from build123d import *

# Parameters (mm, degrees)
SKETCH2_W                     = 76.2
SKETCH2_H                     = 192
BOSS_EXTRUDE1_DEPTH           = 9.525
M16_CLEARANCE_HOLE1_D         = 17
M4X0_7_TAPPED_HOLE1_D         = 3.3
SKETCH9_R                     = 11.5
CUT_EXTRUDE1_DEPTH            = 179.996240317
FILLET1_SIZE                  = 15
M6X1_0_START                  = -94
M6X1_0_TAPPED_HOLE1_OUTLINE_R = 2.5
M6X1_0_TAPPED_HOLE1_DEPTH     = 12


with BuildPart() as part:
    # Sketch2 → Boss-Extrude1 (new body)
    with BuildSketch(Plane(origin=(0, 0, -83.092064992), x_dir=(-1, 0, 0), z_dir=(0, 0, -1))):
        with Locations((10.260528885, 76.076110104)):
            Rectangle(SKETCH2_W, SKETCH2_H)
    extrude(amount=BOSS_EXTRUDE1_DEPTH)

    # M16 Clearance Hole1 (through all)
    with Locations(Plane.XY.offset(-83.092064992)):
        with Locations((-10.260528885, 76.076110104)):
            Hole(M16_CLEARANCE_HOLE1_D / 2)

    # M4x0.7 Tapped Hole1 (through all)
    with Locations(Plane.XY.offset(-83.092064992)):
        with Locations((-21.574237384, 144.762401605), (-26.260528885, 156.076110104), (-21.574237384, 167.389818603), (1.053179614, 144.762401605), (5.739471115, 156.076110104), (1.053179614, 167.389818603), (1.053179614, 7.389818603), (1.053179614, -15.237598395), (-21.574237384, -15.237598395), (-26.260528885, -3.923889896), (-21.574237384, 7.389818603), (5.739471115, -3.923889896)):
            Hole(M4X0_7_TAPPED_HOLE1_D / 2)

    # Sketch9 → Cut-Extrude1 (cut, through all)
    with BuildSketch(Plane.XY.offset(-83.092064992)):
        with Locations((-10.260528885, 156.076110104)):
            Circle(SKETCH9_R)
        with Locations((-10.260528885, -3.923889896)):
            Circle(SKETCH9_R)
    extrude(amount=-CUT_EXTRUDE1_DEPTH, mode=Mode.SUBTRACT)

    # Fillet1
    # a fillet whose section is not a circle: 15 mm, written as the material it takes off along each edge
    with BuildSketch(Plane(origin=(27.839471115, 172.076110104, -45.592064992), x_dir=(0, -1, 0), z_dir=(0, 0, -1)), Plane(origin=(27.839471115, -19.923889896, -45.592064992), x_dir=(-1, 0, 0), z_dir=(0, 0, -1))) as fillet1_piece_1:
        with BuildLine():
            add(Edge.make_bspline([(FILLET1_SIZE, 0), (FILLET1_SIZE * 0.831801948466, 0), (FILLET1_SIZE * 0.663603896932, 0), (FILLET1_SIZE * 0.292893218813, FILLET1_SIZE * 0.0716919198361), (FILLET1_SIZE * 0.0716919198361, FILLET1_SIZE * 0.292893218813), (0, FILLET1_SIZE * 0.663603896932), (0, FILLET1_SIZE * 0.831801948466), (0, FILLET1_SIZE)], knots=[0, 0, 0, 0, 0, 0, 0.5, 0.5, 1, 1, 1, 1, 1, 1], degree=5))
            Line((0, FILLET1_SIZE), (0, 0))
            Line((0, 0), (FILLET1_SIZE, 0))
        make_face()
    extrude(amount=84.525, mode=Mode.SUBTRACT)
    with BuildSketch(Plane(origin=(-48.360528885, -19.923889896, -45.592064992), x_dir=(1, 0, 0), z_dir=(0, 0, -1)), Plane(origin=(-48.360528885, 172.076110104, -45.592064992), x_dir=(0, -1, 0), z_dir=(0, 0, -1))) as fillet1_piece_2:
        with BuildLine():
            add(Edge.make_bspline([(FILLET1_SIZE, 0), (FILLET1_SIZE * 0.831801948466, 0), (FILLET1_SIZE * 0.663603896932, 0), (FILLET1_SIZE * 0.292893218813, -FILLET1_SIZE * 0.0716919198361), (FILLET1_SIZE * 0.0716919198361, -FILLET1_SIZE * 0.292893218813), (0, -FILLET1_SIZE * 0.663603896932), (0, -FILLET1_SIZE * 0.831801948466), (0, -FILLET1_SIZE)], knots=[0, 0, 0, 0, 0, 0, 0.5, 0.5, 1, 1, 1, 1, 1, 1], degree=5))
            Line((0, -FILLET1_SIZE), (0, 0))
            Line((0, 0), (FILLET1_SIZE, 0))
        make_face()
    extrude(amount=84.525, mode=Mode.SUBTRACT)

    # M6x1.0 Tapped Hole1: read off the stored shape, not the designer's step
    # M6x1.0 Tapped Hole1 outline → M6x1.0 Tapped Hole1 (cut)
    with BuildSketch(Plane.XY.offset(M6X1_0_START)):
        with Locations((-30.260528885, 96.076110104)):
            Circle(M6X1_0_TAPPED_HOLE1_OUTLINE_R)
        with Locations((9.739471115, 56.076110104)):
            Circle(M6X1_0_TAPPED_HOLE1_OUTLINE_R)
        with Locations((-30.260528885, 56.076110104)):
            Circle(M6X1_0_TAPPED_HOLE1_OUTLINE_R)
        with Locations((9.739471115, 96.076110104)):
            Circle(M6X1_0_TAPPED_HOLE1_OUTLINE_R)
    extrude(amount=M6X1_0_TAPPED_HOLE1_DEPTH, mode=Mode.SUBTRACT)


solid = part.part
Input: part model. Units: mm. Frame: model coordinates. Coordinates: 2 decimals unless noted, no trailing zeros. Answer in a Markdown table with one row per item. Add a question column.
Item 1: Section query A-A on z = -84.75. State how many separate pieces and enclosed holes the cut face has, then the cut area to 3 significant figures.
Item 2: Contact query for a flat-ended pin moving along its axis: P1, Ø8, axis at x = -30.26, y = 96.08, coming from the -Z side. Output: stop coordinate, or through.
Item 3: Mould query, pull axis X, two halves, no side actions, for faces 1 (the flat face through (-10, -19.924, -88)), 2 (the flat face through (-48.361, 75, -88)), 3 (the cylindrical face through (-23.148, -14.742, -87.921)). Classes: released by +X, released by -X, zero draft, split by the parting line, or undercut.
Item 4: Line query: line 1 along X through (y, z) = (56, -91.25); line 2 along Y through (x, z) = (-30, -92); line 3 along Y through (x, z) = (-3, -90.25). Output: solid intervals per line, ascending. Write a range as [from, to].
Recorded:
| question | item | result |
|---|---|---|
| 1 | separate pieces | 1 |
| 1 | enclosed holes | 19 |
| 1 | area | 13,300 mm^2 |
| 2 | P1 | z = -92.62 |
| 3 | face 1 | zero draft |
| 3 | face 2 | released by -X |
| 3 | face 3 | undercut |
| 4 | line 1 | [-48.36, -32.76], [-27.76, 7.24], [12.24, 27.84] |
| 4 | line 2 | [-19.92, 53.59], [58.56, 93.59], [98.56, 172.08] |
| 4 | line 3 | [-19.92, -12.84], [4.99, 71.66], [80.5, 147.16], [164.99, 172.08] |
